Here's the drawing with two shaded views (mm, measured from the low corner). I have some questions. A direction names the side the tool comes from. Coordinates: 2 decimals unless noted, no trailing zeros. Order: outer loops, then holes, each group sorted by start corner. A loop starts at its lowest first (then second) coordinate and runs counter-clockwise, first axis right, second up. Notation, with made-up numbers: (-26.5, -2) -> (23.5, -2) arc R16 ccw to (23.5, 3) -> close; hole circle Ø3 at (27.5, 76). An arc over 180 degrees is marked (long way). Answer in a Markdown table with one row per item. Add a question column.
1. Imagine slicing it at A-A on y = 45.25. Write out the boundary of the cut face in (x, z), plus the area to 3 significant figures.
2. Imagine slicing it at D-D on x = 11.5. Write out the boundary of the cut face in (y, z).
3. Imagine slicing it at B-B on x = 5.5. Write out the boundary of the cut face in (y, z), plus the area to 3 significant figures.
4. We'd pull the mould along Y, two halves only. Please class the marked faces 6, 7, 8 and 9: pulls with the +Y half, pulls with the -Y half, needs draft (parallel to the pull), parting line crosses it, or undercut.
5. Will these pins go through, and if not, where does the flat tip stop? pin 1 (2.5 mm diameter, centred on x = 5, z = 23, fed in from +Y); pin 2 (6 mm diameter, centred on x = 7, y = 13.5, fed in from +Z); pin 3 (1.5 mm diameter, centred on x = 6, z = 18.5, fed in from +Y); pin 4 (12 mm diameter, centred on y = 41, z = 18.5, fed in from -X).
6. If I drill on line 1 along Z through (x, y) = (15, 0.7); line 2 along Z through (x, y) = (11.45, 17.75); line 3 along X through (y, z) = (45.5, 13), over which ranges is the centre line in solid material (lowest first)? Write a range as [from, to].
7. Imagine slicing it at C-C on z = 5. Write out the boundary of the cut face in (x, y), plus the area to 3 significant figures.
8. On a 3-axis mill with a long thin cutter (end or side, diameter ignored), from which of +Z, -Z, +X, -X, +Y, -Y can I reach the whole of each face in a straight line? I mean the marked faces 1, 2, 3, 4 and 5. Say none if no direction works.
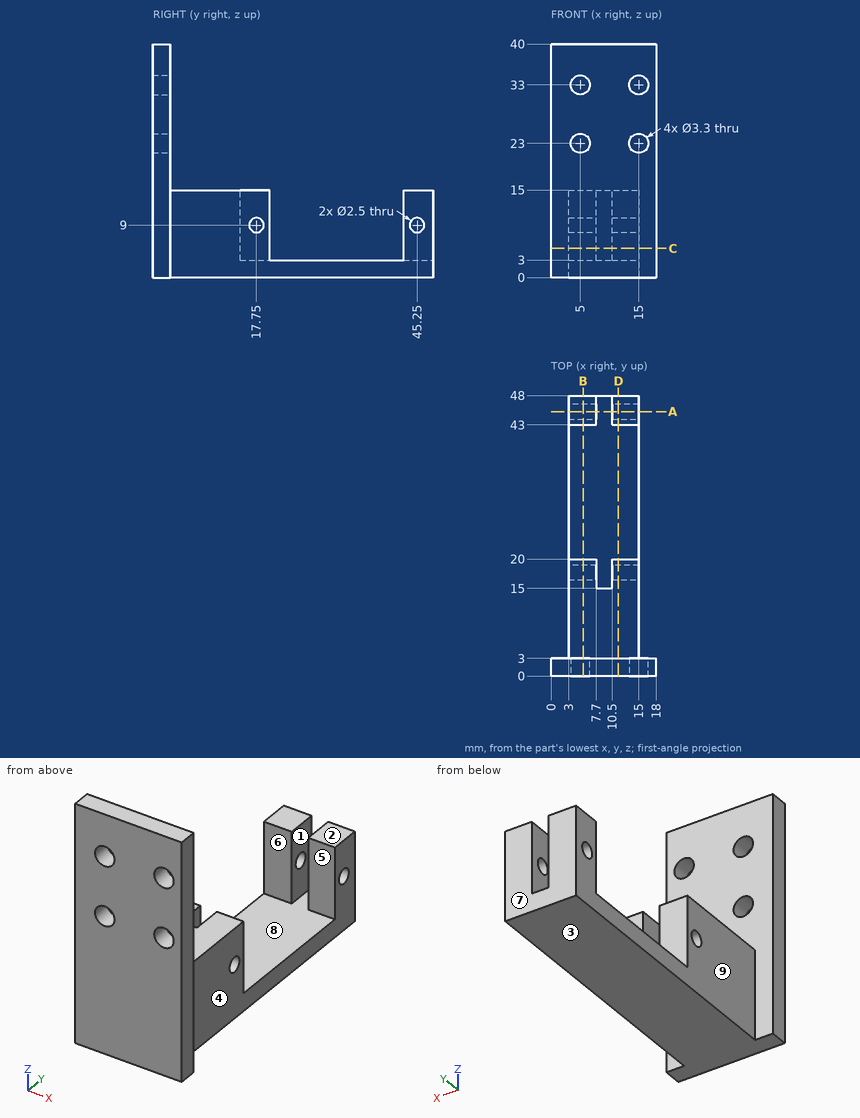
Answers follow:
| question | item | result |
|---|---|---|
| 1 | outline | (3, 0) -> (15, 0) -> (15, 7.75) -> (10.5, 7.75) -> (10.5, 3) -> (7.7, 3) -> (7.7, 7.75) -> (3, 7.75) -> close; (3, 10.25) -> (7.7, 10.25) -> (7.7, 15) -> (3, 15) -> close; (10.5, 10.25) -> (15, 10.25) -> (15, 15) -> (10.5, 15) -> close |
| 1 | area | 123 mm² |
| 2 | outline | (0, 0) -> (48, 0) -> (48, 15) -> (43, 15) -> (43, 3) -> (20, 3) -> (20, 15) -> (3, 15) -> (3, 40) -> (0, 40) -> close; hole circle Ø2.5 at (17.75, 9); hole circle Ø2.5 at (45.25, 9) |
| 3 | outline | (0, 0) -> (48, 0) -> (48, 15) -> (43, 15) -> (43, 3) -> (20, 3) -> (20, 15) -> (3, 15) -> (3, 21.43) -> (0, 21.43) -> close; (0, 24.57) -> (3, 24.57) -> (3, 31.43) -> (0, 31.43) -> close; (0, 34.57) -> (3, 34.57) -> (3, 40) -> (0, 40) -> close; hole circle Ø2.5 at (17.75, 9); hole circle Ø2.5 at (45.25, 9) |
| 3 | area | 490 mm² |
| 4 | face 6 | undercut |
| 4 | face 7 | pulls with the +Y half |
| 4 | face 8 | undercut |
| 4 | face 9 | needs draft |
| 5 | pin 1 | passes through |
| 5 | pin 2 | stops at z = 15 |
| 5 | pin 3 | stops at y = 3 |
| 5 | pin 4 | stops at x = 3 |
| 6 | line 1 | z = [0, 21.35], [24.65, 31.35], [34.65, 40] |
| 6 | line 2 | z = [0, 7.75], [10.25, 15] |
| 6 | line 3 | x = [3, 7.7], [10.5, 15] |
| 7 | outline | (0, 0) -> (18, 0) -> (18, 3) -> (15, 3) -> (15, 20) -> (10.5, 20) -> (10.5, 15) -> (7.7, 15) -> (7.7, 20) -> (3, 20) -> (3, 3) -> (0, 3) -> close; (3, 43) -> (7.7, 43) -> (7.7, 48) -> (3, 48) -> close; (10.5, 43) -> (15, 43) -> (15, 48) -> (10.5, 48) -> close |
| 7 | area | 290 mm² |
| 8 | face 1 | +Z, +Y |
| 8 | face 2 | +Z, +X, -X, +Y |
| 8 | face 3 | -Z, +X, -X, +Y, -Y |
| 8 | face 4 | +Z, -Z, +X, +Y |
| 8 | face 5 | +Z, +X, -X |
